```python
from build123d import *

# Parameters (mm, degrees)
SKETCH1_R           = 2.999999999
SKETCH1_R_2         = 1.5
SKETCH1_R_3         = 1.499999999
BOSS_EXTRUDE1_DEPTH = 5
SKETCH4_R           = 2.5
CUT_EXTRUDE1_DEPTH  = 757.918093325


with BuildPart() as part:
    # Sketch1 → Boss-Extrude1 (new body)
    with BuildSketch(Plane(origin=(0, 0, 0), x_dir=(1, 0, 0), z_dir=(0, 1, 0))):
        with BuildLine():
            Line((40, 0), (510.000000002, 0))
            ThreePointArc((510.000000002, 0), (538.28427125, 11.715728753), (550.000000002, 40))
            Line((550.000000002, 40), (550.000000002, 480))
            ThreePointArc((550.000000002, 480), (538.28427125, 508.284271247), (510.000000002, 520))
            Line((510.000000002, 520), (40, 520))
            ThreePointArc((40, 520), (11.715728753, 508.284271247), (0, 480))
            Line((0, 480), (0, 40))
            ThreePointArc((0, 40), (11.715728753, 11.715728753), (40, 0))
        make_face()
        with Locations(Location((275.000000001, 125, 0), (0, 0, 270))):
            Circle(SKETCH1_R, mode=Mode.SUBTRACT)
        with Locations(Location((200.000000001, 336.45643718, 0), (0, 0, 270))):
            Circle(SKETCH1_R_2, mode=Mode.SUBTRACT)
        with Locations(Location((351.456437186, 336.45643718, 0), (0, 0, 270))):
            Circle(SKETCH1_R_2, mode=Mode.SUBTRACT)
        with Locations(Location((351.456437186, 184.999999996, 0), (0, 0, 270))):
            Circle(SKETCH1_R_2, mode=Mode.SUBTRACT)
        with Locations(Location((200.000000001, 184.999999996, 0), (0, 0, 270))):
            Circle(SKETCH1_R_2, mode=Mode.SUBTRACT)
        with Locations(Location((255.405759863, 113, 0), (0, 0, 270))):
            Circle(SKETCH1_R_2, mode=Mode.SUBTRACT)
        with Locations(Location((210.000000001, 110, 0), (0, 0, 270))):
            Circle(SKETCH1_R_3, mode=Mode.SUBTRACT)
        with Locations(Location((255.405759863, 103, 0), (0, 0, 270))):
            Circle(SKETCH1_R_2, mode=Mode.SUBTRACT)
        with Locations(Location((340.000000001, 140, 0), (0, 0, 270))):
            Circle(SKETCH1_R_3, mode=Mode.SUBTRACT)
        with Locations(Location((210.000000001, 140, 0), (0, 0, 270))):
            Circle(SKETCH1_R_3, mode=Mode.SUBTRACT)
        with Locations(Location((340.000000001, 110, 0), (0, 0, 270))):
            Circle(SKETCH1_R_3, mode=Mode.SUBTRACT)
        Polygon((200.000000001, 326.45643718), (210.000000001, 336.45643718), (340.000000001, 336.45643718), (350.000000001, 326.45643718), (350.000000001, 196.45643718), (340.000000001, 186.45643718), (210.000000001, 186.45643718), (200.000000001, 196.45643718), align=None, mode=Mode.SUBTRACT)
        with BuildLine():
            Line((218.220285237, 120), (218.220285237, 130))
            ThreePointArc((218.220285237, 130), (215.000000001, 133.220285235), (211.779714766, 130))
            Line((211.779714766, 130), (211.779714766, 120))
            ThreePointArc((211.779714766, 120), (215.000000001, 116.779714765), (218.220285237, 120))
        make_face(mode=Mode.SUBTRACT)
    extrude(amount=BOSS_EXTRUDE1_DEPTH)

    # Sketch4 → Cut-Extrude1 (cut, through all)
    with BuildSketch(Plane(origin=(0, 5, 0), x_dir=(1, 0, 0), z_dir=(0, 1, 0))):
        with Locations(Location((535, 70.266316246, 0), (0, 0, 90))):
            Circle(SKETCH4_R)
        with Locations(Location((488.994609259, 10, 0), (0, 0, 90))):
            Circle(SKETCH4_R)
        with Locations(Location((488.994609259, 50, 0), (0, 0, 90))):
            Circle(SKETCH4_R)
        with Locations(Location((535, 100.266316246, 0), (0, 0, 90))):
            Circle(SKETCH4_R)
        with Locations(Location((535, 130.266316246, 0), (0, 0, 90))):
            Circle(SKETCH4_R)
        with Locations(Location((535, 160.266316246, 0), (0, 0, 90))):
            Circle(SKETCH4_R)
        with Locations(Location((535, 190.266316246, 0), (0, 0, 90))):
            Circle(SKETCH4_R)
        with Locations(Location((535, 220.266316246, 0), (0, 0, 90))):
            Circle(SKETCH4_R)
        with Locations(Location((458.994609259, 50, 0), (0, 0, 90))):
            Circle(SKETCH4_R)
        with Locations(Location((458.994609259, 10, 0), (0, 0, 90))):
            Circle(SKETCH4_R)
        with Locations(Location((428.994609259, 50, 0), (0, 0, 90))):
            Circle(SKETCH4_R)
        with Locations(Location((428.994609259, 10, 0), (0, 0, 90))):
            Circle(SKETCH4_R)
        with Locations(Location((398.994609259, 50, 0), (0, 0, 90))):
            Circle(SKETCH4_R)
        with Locations(Location((398.994609259, 10, 0), (0, 0, 90))):
            Circle(SKETCH4_R)
        with Locations(Location((368.994609259, 50, 0), (0, 0, 90))):
            Circle(SKETCH4_R)
        with Locations(Location((368.994609259, 10, 0), (0, 0, 90))):
            Circle(SKETCH4_R)
        with Locations(Location((338.994609259, 50, 0), (0, 0, 90))):
            Circle(SKETCH4_R)
        with Locations(Location((338.994609259, 10, 0), (0, 0, 90))):
            Circle(SKETCH4_R)
        with Locations(Location((338.994609259, 510, 0), (0, 0, 270))):
            Circle(SKETCH4_R)
        with Locations(Location((338.994609259, 470, 0), (0, 0, 270))):
            Circle(SKETCH4_R)
        with Locations(Location((368.994609259, 510, 0), (0, 0, 270))):
            Circle(SKETCH4_R)
        with Locations(Location((368.994609259, 470, 0), (0, 0, 270))):
            Circle(SKETCH4_R)
        with Locations(Location((398.994609259, 510, 0), (0, 0, 270))):
            Circle(SKETCH4_R)
        with Locations(Location((398.994609259, 470, 0), (0, 0, 270))):
            Circle(SKETCH4_R)
        with Locations(Location((428.994609259, 510, 0), (0, 0, 270))):
            Circle(SKETCH4_R)
        with Locations(Location((428.994609259, 470, 0), (0, 0, 270))):
            Circle(SKETCH4_R)
        with Locations(Location((458.994609259, 510, 0), (0, 0, 270))):
            Circle(SKETCH4_R)
        with Locations(Location((458.994609259, 470, 0), (0, 0, 270))):
            Circle(SKETCH4_R)
        with Locations(Location((535, 299.733683754, 0), (0, 0, 270))):
            Circle(SKETCH4_R)
        with Locations(Location((535, 329.733683754, 0), (0, 0, 270))):
            Circle(SKETCH4_R)
        with Locations(Location((535, 359.733683754, 0), (0, 0, 270))):
            Circle(SKETCH4_R)
        with Locations(Location((535, 389.733683754, 0), (0, 0, 270))):
            Circle(SKETCH4_R)
        with Locations(Location((535, 419.733683754, 0), (0, 0, 270))):
            Circle(SKETCH4_R)
        with Locations(Location((488.994609259, 470, 0), (0, 0, 270))):
            Circle(SKETCH4_R)
        with Locations(Location((488.994609259, 510, 0), (0, 0, 270))):
            Circle(SKETCH4_R)
        with Locations(Location((535, 449.733683754, 0), (0, 0, 270))):
            Circle(SKETCH4_R)
        with Locations(Location((211.005390743, 10, 0), (0, 0, 270))):
            Circle(SKETCH4_R)
        with Locations(Location((211.005390743, 50, 0), (0, 0, 270))):
            Circle(SKETCH4_R)
        with Locations(Location((181.005390743, 10, 0), (0, 0, 270))):
            Circle(SKETCH4_R)
        with Locations(Location((181.005390743, 50, 0), (0, 0, 270))):
            Circle(SKETCH4_R)
        with Locations(Location((151.005390743, 10, 0), (0, 0, 270))):
            Circle(SKETCH4_R)
        with Locations(Location((151.005390743, 50, 0), (0, 0, 270))):
            Circle(SKETCH4_R)
        with Locations(Location((121.005390743, 10, 0), (0, 0, 270))):
            Circle(SKETCH4_R)
        with Locations(Location((121.005390743, 50, 0), (0, 0, 270))):
            Circle(SKETCH4_R)
        with Locations(Location((91.005390743, 10, 0), (0, 0, 270))):
            Circle(SKETCH4_R)
        with Locations(Location((91.005390743, 50, 0), (0, 0, 270))):
            Circle(SKETCH4_R)
        with Locations(Location((15.000000002, 220.266316246, 0), (0, 0, 270))):
            Circle(SKETCH4_R)
        with Locations(Location((15.000000002, 190.266316246, 0), (0, 0, 270))):
            Circle(SKETCH4_R)
        with Locations(Location((15.000000002, 160.266316246, 0), (0, 0, 270))):
            Circle(SKETCH4_R)
        with Locations(Location((15.000000002, 130.266316246, 0), (0, 0, 270))):
            Circle(SKETCH4_R)
        with Locations(Location((15.000000002, 100.266316246, 0), (0, 0, 270))):
            Circle(SKETCH4_R)
        with Locations(Location((61.005390743, 50, 0), (0, 0, 270))):
            Circle(SKETCH4_R)
        with Locations(Location((61.005390743, 10, 0), (0, 0, 270))):
            Circle(SKETCH4_R)
        with Locations(Location((15.000000002, 70.266316246, 0), (0, 0, 270))):
            Circle(SKETCH4_R)
        with Locations(Location((15.000000002, 449.733683754, 0), (0, 0, 90))):
            Circle(SKETCH4_R)
        with Locations(Location((61.005390743, 510, 0), (0, 0, 90))):
            Circle(SKETCH4_R)
        with Locations(Location((61.005390743, 470, 0), (0, 0, 90))):
            Circle(SKETCH4_R)
        with Locations(Location((15.000000002, 419.733683754, 0), (0, 0, 90))):
            Circle(SKETCH4_R)
        with Locations(Location((15.000000002, 389.733683754, 0), (0, 0, 90))):
            Circle(SKETCH4_R)
        with Locations(Location((15.000000002, 359.733683754, 0), (0, 0, 90))):
            Circle(SKETCH4_R)
        with Locations(Location((15.000000002, 329.733683754, 0), (0, 0, 90))):
            Circle(SKETCH4_R)
        with Locations(Location((15.000000002, 299.733683754, 0), (0, 0, 90))):
            Circle(SKETCH4_R)
        with Locations(Location((91.005390743, 470, 0), (0, 0, 90))):
            Circle(SKETCH4_R)
        with Locations(Location((91.005390743, 510, 0), (0, 0, 90))):
            Circle(SKETCH4_R)
        with Locations(Location((121.005390743, 470, 0), (0, 0, 90))):
            Circle(SKETCH4_R)
        with Locations(Location((121.005390743, 510, 0), (0, 0, 90))):
            Circle(SKETCH4_R)
        with Locations(Location((151.005390743, 470, 0), (0, 0, 90))):
            Circle(SKETCH4_R)
        with Locations(Location((151.005390743, 510, 0), (0, 0, 90))):
            Circle(SKETCH4_R)
        with Locations(Location((181.005390743, 470, 0), (0, 0, 90))):
            Circle(SKETCH4_R)
        with Locations(Location((181.005390743, 510, 0), (0, 0, 90))):
            Circle(SKETCH4_R)
        with Locations(Location((211.005390743, 470, 0), (0, 0, 90))):
            Circle(SKETCH4_R)
        with Locations(Location((211.005390743, 510, 0), (0, 0, 90))):
            Circle(SKETCH4_R)
    extrude(amount=-CUT_EXTRUDE1_DEPTH, mode=Mode.SUBTRACT)


solid = part.part
```
Geometry check sheet. Reference: the model listing, model coordinates, mm. Round coordinates to 2 decimals unless told otherwise and drop trailing zeros. Use a Markdown table: item, result.
(1) Scan lines: probe 1 along X at (y, z) = (3.35, -109.5); probe 2 along Z at (x, y) = (90.5, 1.6); probe 3 along Z at (x, y) = (225.5, 1.8). Record each from-to range of solid material in increasing order.
Calculated:
| item | result |
|---|---|
| probe 1 | 0 to 208.59, 211.41 to 338.59, 341.41 to 550 |
| probe 2 | -520 to -512.45, -507.55 to -472.45, -467.55 to -52.45, -47.55 to -12.45, -7.55 to 0 |
| probe 3 | -520 to -336.46, -186.46 to 0 |
(2) Go/stop test with a flat-tipped pin: P1, Ø2.5, axis at x = 200, z = -336.46, coming from the +Y side. Record where the tip stops, or that it passes through.
Calculated:
| item | result |
|---|---|
| P1 | through |
(3) Sectioned sample at A-A (y = 3.15). Give the number of separate pieces and of enclosed holes in the cut face, then the cut area to 3 significant figures.
Calculated:
| item | result |
|---|---|
| separate pieces | 1 |
| enclosed holes | 85 |
| area | 261,000 mm² |
